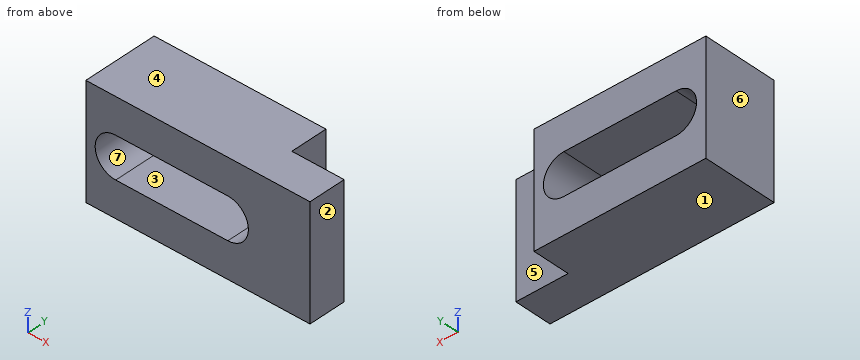
```python
from build123d import *

# Parameters (mm, degrees)
SKETCH1_W               = 30
SKETCH1_H               = 15
BOSS_EXTRUDE1_DEPTH     = 10
CUT_EXTRUDE1_DEPTH      = 24.452078799
CUT_EXTRUDE1_DEPTH_BACK = 24.452078799
SKETCH2_W               = 7
SKETCH2_H               = 5


with BuildPart() as part:
    # Sketch1 → Boss-Extrude1 (new body)
    with BuildSketch(Plane(origin=(0, 0, 0), x_dir=(1, 0, 0), z_dir=(0, 1, 0))):
        Rectangle(SKETCH1_W, SKETCH1_H)
        with BuildLine():
            Line((-11, 2.75), (4, 2.75))
            ThreePointArc((4, 2.75), (6.75, 0), (4, -2.75))
            Line((4, -2.75), (-11, -2.75))
            ThreePointArc((-11, -2.75), (-13.75, 0), (-11, 2.75))
        make_face(mode=Mode.SUBTRACT)
    extrude(amount=BOSS_EXTRUDE1_DEPTH)

    # Sketch2 → Cut-Extrude1 (cut, two sides: drawn at the far end of the back side and taken through both)
    with BuildSketch(Plane.XY.offset(7.5).offset(-CUT_EXTRUDE1_DEPTH_BACK)):
        with Locations((11.5, 7.5)):
            Rectangle(SKETCH2_W, SKETCH2_H)
    extrude(amount=CUT_EXTRUDE1_DEPTH + CUT_EXTRUDE1_DEPTH_BACK, mode=Mode.SUBTRACT)


solid = part.part
```
Part model, mm, in its own coordinate system. Face numbers are marked on the shaded views. A direction names the side the tool comes from. Coordinates: 2 decimals unless noted, no trailing zeros. Order: outer loops, then holes, each group sorted by start corner. A loop starts at its lowest first (then second) coordinate and runs counter-clockwise, first axis right, second up. Notation, with made-up numbers: (55, -38.5) - (61, -38.5) arc R21 ccw to (61, -0.5) - close; hole circle Ø2 at (82, -8.5). An arc over 180 degrees is marked (long way). Return JSON: item names as keys, results as strings. Group by question number.
Item 1: Cut at C-C (y = 2.5). List the corners of the cut face in (x, z), plus the area to 3 significant figures.
Item 2: Which spindle directions (+Z, -Z, +X, -X, +Y, -Y) get a long thin tool onto all of the face, cutting with end or side? Do the marked faces 5, 6 and 7. Say none if no direction does.
Item 3: Pin check, flat tips, straight feed: pin 1 (3 mm diameter, centred on x = 10.5, z = -5.5, fed in from +Y); pin 2 (4 mm diameter, centred on y = 7.5, z = 2, fed in from +X); pin 3 (8 mm diameter, centred on x = 9.5, z = 6, fed in from -Y). Stop position of each tip, or through.
Item 4: Cut at B-B (x = -3.75). List the corners of the cut face in (y, z), plus the area to 3 significant figures.
Item 5: Pull direction Z, two halves, no side cores. Call the marked faces 1, 2, 3 and 4: pulls with the +Z half, pulls with the -Z half, needs draft (parallel to the pull), parting line crosses it, or undercut.
Item 6: Drill centre lines: probe 1 along Z at (x, y) = (-3.75, 6); probe 2 along X at (y, z) = (5.75, 0); probe 3 along Y at (x, z) = (11.5, -1). Where is each one in solid material? Low to high. Write a range as from..to.
Item 7: Cut at D-D (z = -4.75). List the corners of the cut face in (x, y).
Item 8: Cut at A-A (z = 0). List the corners of the cut face in (x, y).
Check values:
{
 "1": {"outline": "(-15, -7.5) - (15, -7.5) - (15, 7.5) - (-15, 7.5) - close; hole (-11, -2.75) - (4, -2.75) arc R2.75 ccw to (4, 2.75) - (-11, 2.75) arc R2.75 ccw to start", "area": "344 mm2"},
 "2": {"face 5": "+Z, -Z, +X, +Y", "face 6": "+Z, -Z, -X, +Y, -Y", "face 7": "+Y, -Y"},
 "3": {"pin 1": "stops at y = 5", "pin 2": "stops at x = 8", "pin 3": "stops at y = 0"},
 "4": {"outline": "(0, -7.5) - (10, -7.5) - (10, -2.75) - (0, -2.75) - close; (0, 2.75) - (10, 2.75) - (10, 7.5) - (0, 7.5) - close", "area": "95.0 mm2"},
 "5": {"face 1": "pulls with the -Z half", "face 2": "needs draft", "face 3": "undercut", "face 4": "pulls with the +Z half"},
 "6": {"probe 1": "z = -7.5..-2.75, 2.75..7.5", "probe 2": "x = -15..-13.75, 6.75..8", "probe 3": "y = 0..5"},
 "7": {"outline": "(-15, 0) - (15, 0) - (15, 5) - (8, 5) - (8, 10) - (-15, 10) - close"},
 "8": {"outline": "(-15, 0) - (-13.75, 0) - (-13.75, 10) - (-15, 10) - close; (6.75, 0) - (15, 0) - (15, 5) - (8, 5) - (8, 10) - (6.75, 10) - close"}
}
